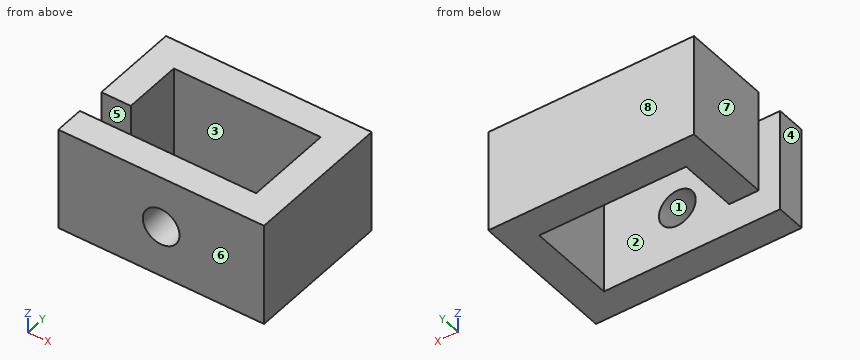
from build123d import *

# Parameters (mm, degrees)
F0_W     = 14
F0_H     = 10
F0_W_2   = 10
F0_H_2   = 6
F1_DEPTH = 7
F2_W     = 2
F2_H     = 2
F3_DEPTH = 10
F4_R     = 1.25
F5_DEPTH = 5


with BuildPart() as f1:
    # F0 (on Top) → F1 (new body)
    with BuildSketch(Plane.XY):
        Rectangle(F0_W, F0_H)
        Rectangle(F0_W_2, F0_H_2, mode=Mode.SUBTRACT)
    extrude(amount=F1_DEPTH)

    # F2 (on face) → F3 (cut)
    with BuildSketch(Plane.XY.offset(7)):
        with Locations((-6, -2)):
            Rectangle(F2_W, F2_H)
    extrude(amount=-F3_DEPTH, mode=Mode.SUBTRACT)

    # F4 (on face) → F5 (cut)
    with BuildSketch(Plane.XZ.offset(5)):
        with Locations((0, 3.5)):
            Circle(F4_R)
    extrude(amount=-F5_DEPTH, mode=Mode.SUBTRACT)


solid = f1.part
For this review, take the finished solid that the model builds, in its own axes (mm). Face numbers are marked on the shaded views. A direction names the side the tool comes from. Give positions to 0.01 mm unless a question says otherwise; leave off trailing zeros. Order: outer loops, then holes, each group sorted by start corner. A loop starts at its lowest first (then second) coordinate and runs counter-clockwise, first axis right, second up. Notation, with made-up numbers: (13.5, -21.5) - (29.5, -21.5) arc R30 ccw to (29.5, 0.5) - close; hole circle Ø1 at (22.5, 65). An arc over 180 degrees is marked (long way). Answer as a JSON object with one key per item and string values. Group by question number.
Item 1: Wall thickness on line 1 along Y through (x, z) = (4.25, 2.75); line 2 along Z through (x, y) = (0, -4.3); line 3 along Y through (x, z) = (-5.25, 3): over which ranges is each line inside the solid? List them lowest first.
Item 2: Take a section at D-D on x = 4.25. Give the boundary of the cut face in (y, z).
Item 3: Machinability: for the marked faces 1, 2, 3 and 4, which of the approach directions +Z, -Z, +X, -X, +Y, -Y give a long, thin tool a straight path to every point of the face, cutting with its end or side? Answer none if there is none.
Item 4: Take a section at C-C on y = 0.25. Give the boundary of the cut face in (x, z).
Item 5: Draft analysis for pull direction Y (two halves, no side actions). For the marked faces 5, 6, 7 and 8, state which applies: pulls with the +Y half, pulls with the -Y half, needs draft (parallel to the pull), parting line crosses it, or undercut.
Item 6: Take a section at B-B on z = 3.5. Give the boundary of the cut face in (x, y), and give its area (3 significant figures).
Item 7: Take a section at A-A on x = 0. Give the boundary of the cut face in (y, z), and give its area (3 significant figures).
Reported:
{
 "1": {"line 1": "-5 to -3, 3 to 5", "line 2": "0 to 2.25, 4.75 to 7", "line 3": "-5 to -3, -1 to 5"},
 "2": {"outline": "(-5, 0) - (-3, 0) - (-3, 7) - (-5, 7) - close; (3, 0) - (5, 0) - (5, 7) - (3, 7) - close"},
 "3": {"face 1": "-Y", "face 2": "+Z, -Z, -X", "face 3": "+Z, -Z", "face 4": "+Z, -Z, -X, +Y, -Y"},
 "4": {"outline": "(-7, 0) - (-5, 0) - (-5, 7) - (-7, 7) - close; (5, 0) - (7, 0) - (7, 7) - (5, 7) - close"},
 "5": {"face 5": "undercut", "face 6": "pulls with the -Y half", "face 7": "needs draft", "face 8": "pulls with the +Y half"},
 "6": {"outline": "(-7, -5) - (-1.25, -5) - (-1.25, -3) - (-7, -3) - close; (-7, -1) - (-5, -1) - (-5, 3) - (5, 3) - (5, -3) - (1.25, -3) - (1.25, -5) - (7, -5) - (7, 5) - (-7, 5) - close", "area": "71.0 mm^2"},
 "7": {"outline": "(-5, 0) - (-3, 0) - (-3, 2.25) - (-5, 2.25) - close; (-5, 4.75) - (-3, 4.75) - (-3, 7) - (-5, 7) - close; (3, 0) - (5, 0) - (5, 7) - (3, 7) - close", "area": "23.0 mm^2"}
}
